Check sheet for the modelled part. Datum: model origin and axes. Units: mm. Give positions to 0.01 mm unless a question says otherwise; leave off trailing zeros. Write each loop counter-clockwise with the first axis right and the second up, starting at its lowest first coordinate (ties: lowest second). Pieces come first, ordered by that corner, then holes. Notation, with made-up numbers: (88.5, 79) -> (104.5, 79) arc R21 ccw to (104.5, 86) -> close; hole circle Ø10 at (-6, 53.5). An arc over 180 degrees is marked (long way). Answer as a JSON object with one key per item and string values.
from build123d import *
from OCP.BRepFilletAPI import BRepFilletAPI_MakeChamfer

# Parameters (mm, degrees)
SKETCH1_R           = 22.5
SKETCH1_R_2         = 4
SKETCH1_R_3         = 1.89865
SKETCH1_R_4         = 1.5875
BOSS_EXTRUDE1_DEPTH = 6.35
CHAMFER1_SIZE       = 2.301024407
CHAMFER1_SIZE2      = 2.00025


with BuildPart() as part:
    # Sketch1 → Boss-Extrude1 (new body)
    with BuildSketch(Plane.XY):
        Circle(SKETCH1_R)
        Circle(SKETCH1_R_2, mode=Mode.SUBTRACT)
        with Locations((0, 15)):
            Circle(SKETCH1_R_3, mode=Mode.SUBTRACT)
        with Locations((10.606601718, 10.606601718)):
            Circle(SKETCH1_R_4, mode=Mode.SUBTRACT)
        with Locations((15, 0)):
            Circle(SKETCH1_R_3, mode=Mode.SUBTRACT)
        with Locations((10.606601718, -10.606601718)):
            Circle(SKETCH1_R_4, mode=Mode.SUBTRACT)
        with Locations((0, -15)):
            Circle(SKETCH1_R_3, mode=Mode.SUBTRACT)
        with Locations((-10.606601718, -10.606601718)):
            Circle(SKETCH1_R_4, mode=Mode.SUBTRACT)
        with Locations((-15, 0)):
            Circle(SKETCH1_R_3, mode=Mode.SUBTRACT)
        with Locations((-10.606601718, 10.606601718)):
            Circle(SKETCH1_R_4, mode=Mode.SUBTRACT)
    extrude(amount=BOSS_EXTRUDE1_DEPTH)

    # Chamfer1: one chamfer whose edges measure the first distance from different faces: ONE call of the kernel's chamfer builder (chamfer() names one face for all edges)
    chamfer1_edges_1 = [part.edges().sort_by_distance(p)[0] for p in [
        (13.10135, 0, 6.35),
    ]]
    chamfer1_side_1 = [part.faces().sort_by_distance(p)[0] for p in [
        (13.10135, 0, 3.175),
    ]]
    chamfer1_edges_2 = [part.edges().sort_by_distance(p)[0] for p in [
        (-1.89865, -15, 6.35),
    ]]
    chamfer1_side_2 = [part.faces().sort_by_distance(p)[0] for p in [
        (-1.89865, -15, 3.175),
    ]]
    chamfer1_edges_3 = [part.edges().sort_by_distance(p)[0] for p in [
        (-16.89865, 0, 6.35),
    ]]
    chamfer1_side_3 = [part.faces().sort_by_distance(p)[0] for p in [
        (-16.89865, 0, 3.175),
    ]]
    chamfer1_edges_4 = [part.edges().sort_by_distance(p)[0] for p in [
        (-1.89865, 15, 6.35),
    ]]
    chamfer1_side_4 = [part.faces().sort_by_distance(p)[0] for p in [
        (-1.89865, 15, 3.175),
    ]]
    chamfer1 = BRepFilletAPI_MakeChamfer(part.part.solid().wrapped)
    for e in chamfer1_edges_1:
        chamfer1.Add(CHAMFER1_SIZE, CHAMFER1_SIZE2, e.wrapped, chamfer1_side_1[0].wrapped)  # the first distance lies on this face
    for e in chamfer1_edges_2:
        chamfer1.Add(CHAMFER1_SIZE, CHAMFER1_SIZE2, e.wrapped, chamfer1_side_2[0].wrapped)  # the first distance lies on this face
    for e in chamfer1_edges_3:
        chamfer1.Add(CHAMFER1_SIZE, CHAMFER1_SIZE2, e.wrapped, chamfer1_side_3[0].wrapped)  # the first distance lies on this face
    for e in chamfer1_edges_4:
        chamfer1.Add(CHAMFER1_SIZE, CHAMFER1_SIZE2, e.wrapped, chamfer1_side_4[0].wrapped)  # the first distance lies on this face
    add(Compound.cast(chamfer1.Shape()), mode=Mode.REPLACE)


solid = part.part
1. Scan lines: L1, parallel to Y at x = 0, z = 3.25; L2, parallel to Y at x = 9.5, z = 1.75; L3, parallel to Y at x = 10, z = 3.75. Record each from-to range of solid material in increasing order. Write a range as [from, to].
Determined:
{"L1": "[-22.5, -16.9], [-13.1, -4], [4, 13.1], [16.9, 22.5]", "L2": "[-20.4, -11.74], [-9.47, 9.47], [11.74, 20.4]", "L3": "[-20.16, -12.07], [-9.14, 9.14], [12.07, 20.16]"}
2. Sectioned sample at C-C, the plane y = -15. Enter the section's corners in (x, z).
Determined:
{"outline": "(-16.77, 0) -> (-1.9, 0) -> (-1.9, 4.05) -> (-3.9, 6.35) -> (-16.77, 6.35) -> close; (1.9, 0) -> (16.77, 0) -> (16.77, 6.35) -> (3.9, 6.35) -> (1.9, 4.05) -> close"}
3. Go/stop test with a flat-tipped pin: P1, Ø1.9, axis at x = -10.61, y = 10.61, coming from the -Z side. Record where the tip stops, or that it passes through.
Determined:
{"P1": "through"}
4. Sectioned sample at B-B, the plane z = 5.5. State how many separate pieces and enclosed holes the cut face has, plus the area to 3 significant figures.
Determined:
{"separate pieces": "1", "enclosed holes": "9", "area": "1,380 mm^2"}
5. Sectioned sample at A-A, the plane x = 0. Enter the section's corners in (y, z), plus the area to 3 significant figures.
Determined:
{"outline": "(-22.5, 0) -> (-16.9, 0) -> (-16.9, 4.05) -> (-18.9, 6.35) -> (-22.5, 6.35) -> close; (-13.1, 0) -> (-4, 0) -> (-4, 6.35) -> (-11.1, 6.35) -> (-13.1, 4.05) -> close; (4, 0) -> (13.1, 0) -> (13.1, 4.05) -> (11.1, 6.35) -> (4, 6.35) -> close; (16.9, 0) -> (22.5, 0) -> (22.5, 6.35) -> (18.9, 6.35) -> (16.9, 4.05) -> close", "area": "178 mm^2"}
6. Mould release check, pull along X, two halves, no side actions. Record for faces 1 (the face through (0, -5, 6.35)), 2 (the face through (-1.492, 16.368, 4.193)), 3 (the face through (10.382, -19.961, 3.131)): released by +X, released by -X, zero draft, split by the parting line, or undercut.
Determined:
{"face 1": "zero draft", "face 2": "undercut", "face 3": "split by the parting line"}
